Here's how the part is built. I have some questions about the finished solid (model axes, mm). A direction names the side the tool comes from. Coordinates: 2 decimals unless noted, no trailing zeros. Order: outer loops, then holes, each group sorted by start corner. A loop starts at its lowest first (then second) coordinate and runs counter-clockwise, first axis right, second up. Notation, with made-up numbers: (78.25, 0) - (99.25, 0) arc R21 ccw to (99.25, 20) - close; hole circle Ø6 at (83, -36). An arc over 180 degrees is marked (long way). Answer as CSV lines item,"result". Start each with the question number.
Q1. Suppose I cut it at C-C (x = 15). Please give me the cut outline in (y, z).
Q2. Suppose I cut it at A-A (z = 3.5). Please give me the cut outline in (x, y).
Q3. For pin 1 Ø2 at (x, y) = (-2, 0) entering from +Z; pin 2 Ø6 at (x, y) = (-16.5, 2.5) entering from -Z, each with a flat end and sliding along its axis, tell me the tip position at first contact or that it passes through.
Q4. Suppose I cut it at D-D (y = 2.5). Please give me the cut outline in (x, z), then the cut area to 3 significant figures.
Q5. I need wall thicknesses on line 1 (X direction, y = -0.25, z = 7.75); line 2 (Y direction, x = 21.5, z = 1.5); line 3 (X direction, y = 0.75, z = 2.5). Which ranges of each line are inside material? Lowest first, please.
Q6. For faces 1 (the face through (7, 0, 9)), 2 (the face through (0, -3.16, 3)), 3 (the face through (8.715, 6.049, 8.592)), which set-ups out of +Z, -Z, +X, -X, +Y, -Y let a thin tool reach every point of the face, with its end or its side?
Q7. Suppose I cut it at B-B (z = 9). Count the separate pieces of the cut face and the enclosed holes in it, then the cut area to 3 significant figures.
from build123d import *

# Parameters (mm, degrees)
SKETCH1_W           = 50
SKETCH1_H           = 12.7
BOSS_EXTRUDE1_DEPTH = 6.55
SKETCH2_W           = 48
SKETCH2_H           = 6.32
CUT_EXTRUDE2_DEPTH  = 6.35
SKETCH3_W           = 2
SKETCH3_H           = 12.7
BOSS_EXTRUDE2_DEPTH = 5
LPATTERN1_COUNT     = 4
LPATTERN1_PITCH     = 16
FILLET1_R           = 1


with BuildPart() as part:
    # Sketch1 → Boss-Extrude1 (new body)
    with BuildSketch(Plane.XY):
        Rectangle(SKETCH1_W, SKETCH1_H)
    extrude(amount=BOSS_EXTRUDE1_DEPTH)

    # Sketch2 → Cut-Extrude2 (cut)
    with BuildSketch(Plane(origin=(0, 0, 0), x_dir=(-1, 0, 0), z_dir=(0, 0, -1))):
        Rectangle(SKETCH2_W, SKETCH2_H)
    extrude(amount=-CUT_EXTRUDE2_DEPTH, mode=Mode.SUBTRACT)

    # Sketch3 → Boss-Extrude2 (add)
    with BuildSketch(Plane.XY.offset(6.55)):
        with Locations((-24, 0)):
            Rectangle(SKETCH3_W, SKETCH3_H)
    boss_extrude2 = extrude(amount=BOSS_EXTRUDE2_DEPTH)

    # LPattern1: Boss-Extrude2 ×4
    with Locations(*[(i * LPATTERN1_PITCH, 0, 0) for i in range(1, LPATTERN1_COUNT)]):
        add(boss_extrude2)

    # Fillet1
    fillet1_edges = [part.edges().sort_by_distance(p)[0] for p in [
        (-16, -6.35, 6.55),
        (-23, -6.35, 9.05),
        (-23, 6.35, 9.05),
        (-24, -6.35, 11.55),
        (-24, 6.35, 11.55),
        (0, -6.35, 6.55),
        (-16, 6.35, 6.55),
        (-9, 6.35, 9.05),
        (-9, -6.35, 9.05),
        (-7, -6.35, 9.05),
        (-7, 6.35, 9.05),
        (-8, -6.35, 11.55),
        (-8, 6.35, 11.55),
        (0, 6.35, 0),
        (0, 6.35, 6.55),
        (16, -6.35, 6.55),
        (7, 6.35, 9.05),
        (7, -6.35, 9.05),
        (9, -6.35, 9.05),
        (9, 6.35, 9.05),
        (8, -6.35, 11.55),
        (8, 6.35, 11.55),
        (0, -6.35, 0),
        (16, 6.35, 6.55),
        (23, 6.35, 9.05),
        (23, -6.35, 9.05),
        (24, -6.35, 11.55),
        (24, 6.35, 11.55),
        (-25, 6.35, 5.775),
        (25, 6.35, 5.775),
        (25, -6.35, 5.775),
        (-25, -6.35, 5.775),
    ]]
    fillet(fillet1_edges, radius=FILLET1_R - 0.0001)  # a hair under: the kernel refuses the full size


solid = part.part
Here are the results:
1,outline,"(-6.35, 1) arc R1 ccw to (-5.35, 0) - (-3.16, 0) - (-3.16, 6.35) - (3.16, 6.35) - (3.16, 0) - (5.35, 0) arc R1 ccw to (6.35, 1) - (6.35, 5.55) arc R1 ccw to (5.35, 6.55) - (-5.35, 6.55) arc R1 ccw to (-6.35, 5.55) - close"
2,outline,"(-25, -5.35) arc R1 ccw to (-24, -6.35) - (24, -6.35) arc R1 ccw to (25, -5.35) - (25, 5.35) arc R1 ccw to (24, 6.35) - (-24, 6.35) arc R1 ccw to (-25, 5.35) - close; hole (-24, -3.16) - (24, -3.16) - (24, 3.16) - (-24, 3.16) - close"
3,pin 1,"stops at z = 6.55"
3,pin 2,"stops at z = 0"
4,outline,"(-25, 0) - (-24, 0) - (-24, 6.35) - (24, 6.35) - (24, 0) - (25, 0) - (25, 11.55) - (23, 11.55) - (23, 6.55) - (9, 6.55) - (9, 11.55) - (7, 11.55) - (7, 6.55) - (-7, 6.55) - (-7, 11.55) - (-9, 11.55) - (-9, 6.55) - (-23, 6.55) - (-23, 11.55) - (-25, 11.55) - close"
4,area,"62.7 mm²"
5,line 1,"x = -25 to -23, -9 to -7, 7 to 9, 23 to 25"
5,line 2,"y = -6.35 to -3.16, 3.16 to 6.35"
5,line 3,"x = -25 to -24, 24 to 25"
6,face 1,"+Z, +Y, -Y"
6,face 2,"-Z"
6,face 3,"+Z, +Y"
7,separate pieces,"4"
7,enclosed holes,"0"
7,area,"98.2 mm²"
